```python
from build123d import *

# Parameters (mm, degrees)
ESQUISSE1_R                  = 32.5
BOSS_EXTRU_1_DEPTH           = 12
ESQUISSE2_R                  = 28
ESQUISSE2_R_2                = 8
ENL_V_MAT_EXTRU_1_DEPTH      = 4
CHANFREIN1_SIZE              = 4
CHANFREIN2_SIZE              = 2
CHANFREIN1_OF_SYM_TRIE1_SIZE = 4
CHANFREIN2_OF_SYM_TRIE1_SIZE = 2


with BuildPart() as part:
    # Esquisse1 → Boss.-Extru.1 (new body)
    with BuildSketch(Plane.XY):
        Circle(ESQUISSE1_R)
        with BuildLine():
            Line((-1.354529956, 1.471478372), (1.732143973, 0.999838616))
            ThreePointArc((1.732143973, 0.999838616), (-0.302091213, -1.97705359), (-1.354529956, 1.471478372))
        make_face(mode=Mode.SUBTRACT)
        with BuildLine():
            ThreePointArc((-10.724622204, 8.999026536), (-5.916655664, 12.688309019), (0, 14))
            ThreePointArc((0, 14), (4, 18), (0, 22))
            ThreePointArc((0, 22), (-9.297601758, 19.938771315), (-16.852977749, 14.141327413))
            ThreePointArc((-16.852977749, 14.141327413), (-16.359950415, 8.505999202), (-10.724622204, 8.999026536))
        make_face(mode=Mode.SUBTRACT)
        with BuildLine():
            ThreePointArc((22, 0), (19.938771315, 9.297601758), (14.141327413, 16.852977749))
            ThreePointArc((14.141327413, 16.852977749), (8.505999202, 16.359950415), (8.999026536, 10.724622204))
            ThreePointArc((8.999026536, 10.724622204), (12.688309019, 5.916655664), (14, 0))
            ThreePointArc((14, 0), (18, -4), (22, 0))
        make_face(mode=Mode.SUBTRACT)
        with BuildLine():
            ThreePointArc((0, -22), (9.297601758, -19.938771315), (16.852977749, -14.141327413))
            ThreePointArc((16.852977749, -14.141327413), (16.359950415, -8.505999202), (10.724622204, -8.999026536))
            ThreePointArc((10.724622204, -8.999026536), (5.916655664, -12.688309019), (0, -14))
            ThreePointArc((0, -14), (-4, -18), (0, -22))
        make_face(mode=Mode.SUBTRACT)
        with BuildLine():
            ThreePointArc((-22, 0), (-19.938771315, -9.297601758), (-14.141327413, -16.852977749))
            ThreePointArc((-14.141327413, -16.852977749), (-8.505999202, -16.359950415), (-8.999026536, -10.724622204))
            ThreePointArc((-8.999026536, -10.724622204), (-12.688309019, -5.916655664), (-14, 0))
            ThreePointArc((-14, 0), (-18, 4), (-22, 0))
        make_face(mode=Mode.SUBTRACT)
    extrude(amount=BOSS_EXTRU_1_DEPTH)

    # Esquisse2 → Enlèv. mat.-Extru.1 (cut)
    with BuildSketch(Plane.XY.offset(12)):
        Circle(ESQUISSE2_R)
        Circle(ESQUISSE2_R_2, mode=Mode.SUBTRACT)
    enl_v_mat_extru_1 = extrude(amount=-ENL_V_MAT_EXTRU_1_DEPTH, mode=Mode.SUBTRACT)

    # Chanfrein1
    chanfrein1_edges = [part.edges().sort_by_distance(p)[0] for p in [
        (-8, 0, 8),
    ]]
    chamfer(chanfrein1_edges, length=CHANFREIN1_SIZE - 0.0001)  # a hair under: the kernel refuses the full size

    # Chanfrein2
    chanfrein2_edges = [part.edges().sort_by_distance(p)[0] for p in [
        (-28, 0, 8),
    ]]
    chamfer(chanfrein2_edges, length=CHANFREIN2_SIZE)

    # Symétrie1: Enlèv. mat.-Extru.1 across plane
    add(enl_v_mat_extru_1.mirror(Plane.XY.offset(6)), mode=Mode.SUBTRACT)

    # Chanfrein1 of Symétrie1
    chanfrein1_of_sym_trie1_edges = [part.edges().sort_by_distance(p)[0] for p in [
        (-8, 0, 4),
    ]]
    chamfer(chanfrein1_of_sym_trie1_edges, length=CHANFREIN1_OF_SYM_TRIE1_SIZE - 0.0001)  # a hair under: the kernel refuses the full size

    # Chanfrein2 of Symétrie1
    chanfrein2_of_sym_trie1_edges = [part.edges().sort_by_distance(p)[0] for p in [
        (-28, 0, 4),
    ]]
    chamfer(chanfrein2_of_sym_trie1_edges, length=CHANFREIN2_OF_SYM_TRIE1_SIZE)


solid = part.part
```
Build history of the part. All positions in model axes, mm. A direction names the side the tool comes from. Give positions to 0.01 mm unless a question says otherwise; leave off trailing zeros. One line per question, with ' | ' between items. Start each with the question number.
1) Cut at A-A (y = 2.5). Count the separate pieces of the cut face and the enclosed holes in it, plus the area to 3 significant figures.
2) Two-plate mould, pull along X, no slides. Class faces 5 (the cylindrical face through (31, 9.76, 5.92)), 6 (the flat face through (9, 27, 0)), 7 (the cylindrical face through (0, -2, 6)): released by +X, released by -X, zero draft, split by the parting line, or undercut.
3) Probe L1, parallel to Y at x = 11.5, z = 5 (3 decimals); L2, parallel to Y at x = 0, z = 1.45; L3, parallel to X at y = -1, z = 2.75. List the from-to ranges inside material, lowest first.
4) Pin check, flat tips, straight feed: pin 1 (2 mm diameter, centred on x = -6.5, z = 7, fed in from -Y); pin 2 (1.5 mm diameter, centred on x = 4, y = -8, fed in from +Z); pin 3 (1.5 mm diameter, centred on x = -10, z = 3, fed in from -Y); pin 4 (4.5 mm diameter, centred on x = 0, y = 0, fed in from +Z). Stop position of each tip, or through.
5) 3-axis set-ups, long thin cutter, end or side, ignore diameter. For faces 1 (the flat face through (11.2, -5.4, 8)), 2 (the cylindrical face through (-19.995, -9.176, 5.972)), 3 (the flat face through (0, 2, 0)), 4 (the flat face through (11.2, -5.4, 4)): which of +Z, -Z, +X, -X, +Y, -Y reach the whole face in a straight line?
Return value:
1) separate pieces: 3 | enclosed holes: 0 | area: 437 mm^2
2) face 5: split by the parting line | face 6: zero draft | face 7: undercut
3) L1: -30.397 to -18.755, -8.29 to 7.984, 17.788 to 30.397 | L2: -32.5 to -28, -9.45 to -2, 1.26 to 9.45, 28 to 32.5 | L3: -32.48 to -27.23, -10.7 to -1.73, 1.73 to 10.7, 27.23 to 32.48
4) pin 1: y = -32.03 | pin 2: z = 11.81 | pin 3: y = -31.16 | pin 4: z = 12
5) face 1: +Z | face 2: +Z, -Z | face 3: -Z, +X, -X, +Y, -Y | face 4: -Z
